Verification items for the finished model (mm, model axes). Coordinates: 2 decimals unless noted, no trailing zeros. Write each loop counter-clockwise with the first axis right and the second up, starting at its lowest first coordinate (ties: lowest second). Pieces come first, ordered by that corner, then holes. Notation, with made-up numbers: M -26.75,25 L 10.25,25 A8 cw 10.25,36 Z; hole C 9,-7 d9. An arc over 180 degrees is marked long. Answer in a Markdown table with one row per item.
from build123d import *

# Parameters (mm, degrees)
CROQUIS1_R              = 6.35
SALIENTE_EXTRUIR1_DEPTH = 10


with BuildPart() as part:
    # Croquis1 → Saliente-Extruir1 (new body)
    with BuildSketch(Plane(origin=(0, 0, 0), x_dir=(1, 0, 0), z_dir=(0, 1, 0))):
        Polygon((-7.332348419, -12.7), (7.332348419, -12.7), (14.664696837, 0), (7.332348419, 12.7), (-7.332348419, 12.7), (-14.664696837, 0), align=None)
        Circle(CROQUIS1_R, mode=Mode.SUBTRACT)
    extrude(amount=SALIENTE_EXTRUIR1_DEPTH)

    # Croquis2 → Cortar-Revolución1 (revolve, cut)
    with BuildSketch(Plane.XY):
        Polygon((-14.664696837, 8), (-12.664696837, 10), (-14.664696837, 10), align=None)
    cortar_revoluci_n1 = revolve(axis=Axis((0, 0, 0), (0, 1, 0)), mode=Mode.SUBTRACT)

    # Simetría1: Cortar-Revolución1 across plane
    add(cortar_revoluci_n1.mirror(Plane.ZX.offset(5)), mode=Mode.SUBTRACT)


solid = part.part
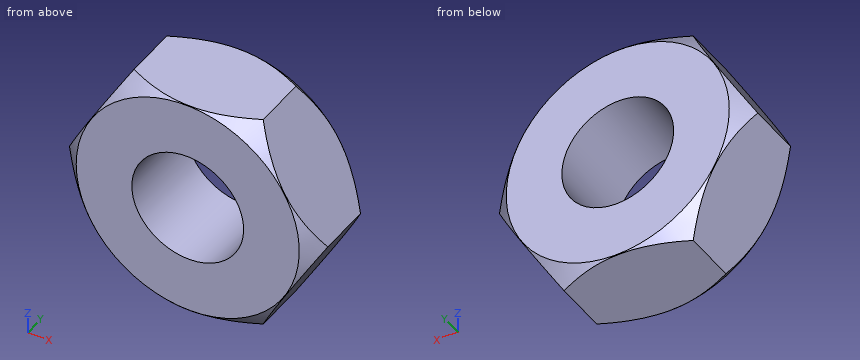
1) Sectioned sample at C-C (y = 8.75). Record the cut outline in (x, z).
Response values:
| item | result |
|---|---|
| outline | M -13.84,-1.43 L -8.16,-11.27 A13.91 ccw -5.69,-12.7 L 5.69,-12.7 A13.91 ccw 8.16,-11.27 L 13.84,-1.43 A13.91 ccw 13.84,1.43 L 8.16,11.27 A13.91 ccw 5.69,12.7 L -5.69,12.7 A13.91 ccw -8.16,11.27 L -13.84,1.43 A13.91 ccw Z; hole C 0,0 d12.7 |
2) Depth check by flat-ended pin: pin 1 (11.5 mm diameter, centred on x = 0, z = 0, fed in from -Y); pin 2 (2 mm diameter, centred on x = -9.5, z = -6, fed in from -Y). Enter the tip coordinate at first touch or a pass-through.
Response values:
| item | result |
|---|---|
| pin 1 | passes through |
| pin 2 | stops at y = 0 |
3) Sectioned sample at A-A (x = 0). Record the cut outline in (y, z).
Response values:
| item | result |
|---|---|
| outline | M 0,-12.66 L 0.04,-12.7 L 9.96,-12.7 L 10,-12.66 L 10,-6.35 L 0,-6.35 Z; M 0,6.35 L 10,6.35 L 10,12.66 L 9.96,12.7 L 0.04,12.7 L 0,12.66 Z |
4) Sectioned sample at B-B (y = 3.5). Record the cut outline in (x, z), then the cut area to 3 significant figures.
Response values:
| item | result |
|---|---|
| outline | M -14.66,0 L -7.33,-12.7 L 7.33,-12.7 L 14.66,0 L 7.33,12.7 L -7.33,12.7 Z; hole C 0,0 d12.7 |
| area | 432 mm² |
5) Thickness scan on L1, parallel to Z at x = 0, y = 6; L2, parallel to X at y = 1, z = 5.75; L3, parallel to Z at x = 2.25, y = 7. Record the ranges inside material, lowest first. Write a range as [from, to].
Response values:
| item | result |
|---|---|
| L1 | z = [-12.7, -6.35], [6.35, 12.7] |
| L2 | x = [-11.34, -2.69], [2.69, 11.34] |
| L3 | z = [-12.7, -5.94], [5.94, 12.7] |
